Check sheet for the modelled part. Datum: model origin and axes. Units: mm. A direction names the side the tool comes from. Coordinates: 2 decimals unless noted, no trailing zeros. Write each loop counter-clockwise with the first axis right and the second up, starting at its lowest first coordinate (ties: lowest second). Pieces come first, ordered by that corner, then holes. Notation, with made-up numbers: (69.25, 21.5) -> (81.25, 21.5) arc R33 ccw to (81.25, 53.5) -> close; hole circle Ø3 at (24, 64). An arc over 180 degrees is marked (long way). One line per item, written item: value. Start each with the question number.
1) Sectioned sample at A-A on y = 9. Enter the section's corners in (x, z).
2) Scan lines: line 1 along Y through (x, z) = (0, 0.75); line 2 along X through (y, z) = (9, 1.5); line 3 along X through (y, z) = (7.75, 3.25). Record each from-to range of solid material in increasing order. Write a range as [from, to].
3) Sectioned sample at B-B on x = 0. Enter the section's corners in (y, z), plus the area to 3 significant figures.
4) Gauge pin test, flat ends, axial feed: P1, Ø1.3, axis at x = 4, y = 5, coming from the +Z side; P2, Ø5.5, axis at x = 0, y = 9, coming from the -Z side; P3, Ø1.1, axis at y = 8.5, z = 4, coming from the +X side. Record the tip position at first contact, or that the pin passes through.
5) Draft check along Y on faces 4 (the cylindrical face through (0.273, 11.082, 0.852)), 5 (the flat face through (0, 0, 1)), 6 (the flat face through (-3.5, 8.9, -1)), 7 (the flat face through (0, 18, 1)). Enter one of: +Y half, -Y half, draft (parallel to the pull), parting line (faces both ways), or undercut.
6) Sectioned sample at C-C on z = 3. Enter the section's corners in (x, y).
7) Set-up check for faces 1 (the flat face through (3.4, 8.9, -1.1)), 2 (the flat face through (2.9, 9, 3)), 3 (the flat face through (-2.9, 9, 3)): record each of +Z, -Z, +X, -X, +Y, -Y from which the full face is reachable in a straight line by a thin tool's end or side.
8) Sectioned sample at D-D on y = 15. Enter the section's corners in (x, z).
```python
from build123d import *

# Parameters (mm, degrees)
EXTRUDE_1_DEPTH    = 18
CHAMFER_1_SIZE     = 3
CHAMFER_2_SIZE     = 0.2
HOLE_WIZARD_M5_1_D = 4.2


with BuildPart() as part:
    # 草图1 → 凸台-拉伸1 (new body)
    with BuildSketch(Plane(origin=(0, 0, 0), x_dir=(1, 0, 0), z_dir=(0, 1, 0))):
        Polygon((2.9, -2.55), (4.95, -2.55), (4.95, 2.55), (-4.95, 2.55), (-4.95, -2.55), (-2.9, -2.55), (-2.9, -4.35), (2.9, -4.35), align=None)
    extrude(amount=EXTRUDE_1_DEPTH)

    # 倒角1
    chamfer_1_edges = [part.edges().sort_by_distance(p)[0] for p in [
        (-4.95, 9, -2.55),
        (4.95, 9, -2.55),
    ]]
    chamfer(chamfer_1_edges, length=CHAMFER_1_SIZE)

    # 倒角2
    chamfer_2_edges = [part.edges().sort_by_distance(p)[0] for p in [
        (4.95, 9, 2.55),
        (2.9, 9, 2.55),
        (2.9, 9, 4.35),
        (-2.9, 9, 4.35),
        (-2.9, 9, 2.55),
        (-4.95, 9, 2.55),
    ]]
    chamfer(chamfer_2_edges, length=CHAMFER_2_SIZE)

    # M5 螺纹孔1 (through all)
    with Locations(Plane.XY.offset(4.35)):
        with Locations((0, 9)):
            Hole(HOLE_WIZARD_M5_1_D / 2)


solid = part.part
```
Answers:
1. outline: (-4.95, 0.45) -> (-2.1, -2.4) -> (-2.1, 4.35) -> (-2.7, 4.35) -> (-2.9, 4.15) -> (-2.9, 2.75) -> (-3.1, 2.55) -> (-4.75, 2.55) -> (-4.95, 2.35) -> close; (2.1, -2.4) -> (4.95, 0.45) -> (4.95, 2.35) -> (4.75, 2.55) -> (3.1, 2.55) -> (2.9, 2.75) -> (2.9, 4.15) -> (2.7, 4.35) -> (2.1, 4.35) -> close
2. line 1: y = [0, 6.9], [11.1, 18]
2. line 2: x = [-4.95, -2.1], [2.1, 4.95]
2. line 3: x = [-2.9, -1.69], [1.69, 2.9]
3. outline: (0, -2.55) -> (6.9, -2.55) -> (6.9, 4.35) -> (0, 4.35) -> close; (11.1, -2.55) -> (18, -2.55) -> (18, 4.35) -> (11.1, 4.35) -> close
3. area: 95.2 mm2
4. P1: stops at z = 2.55
4. P2: stops at z = -2.55
4. P3: stops at x = 2.9
5. face 4: undercut
5. face 5: -Y half
5. face 6: draft
5. face 7: +Y half
6. outline: (-2.9, 0) -> (2.9, 0) -> (2.9, 18) -> (-2.9, 18) -> close; hole circle Ø4.2 at (0, 9)
7. face 1: -Z, +X, +Y, -Y
7. face 2: +Z, +X, +Y, -Y
7. face 3: +Z, -X, +Y, -Y
8. outline: (-4.95, 0.45) -> (-1.95, -2.55) -> (1.95, -2.55) -> (4.95, 0.45) -> (4.95, 2.35) -> (4.75, 2.55) -> (3.1, 2.55) -> (2.9, 2.75) -> (2.9, 4.15) -> (2.7, 4.35) -> (-2.7, 4.35) -> (-2.9, 4.15) -> (-2.9, 2.75) -> (-3.1, 2.55) -> (-4.75, 2.55) -> (-4.95, 2.35) -> close
